```python
from build123d import *

# Parameters (mm, degrees)
ESBO_O1_W                = 22
ESBO_O1_H                = 36
RESSALTO_EXTRUS_O1_DEPTH = 110
CASCA1_T                 = -2
ESBO_O2_R                = 5
CORTE_EXTRUS_O1_DEPTH    = 1000
ESBO_O3_R                = 2.75
CORTE_EXTRUS_O2_DEPTH    = 29


with BuildPart() as part:
    # Esboço1 → Ressalto-extrusão1 (new body)
    with BuildSketch(Plane.XY):
        with Locations((0, 18)):
            Rectangle(ESBO_O1_W, ESBO_O1_H)
    extrude(amount=RESSALTO_EXTRUS_O1_DEPTH)

    # Casca1
    casca1_openings = [part.faces().sort_by_distance(p)[0] for p in [
        (0, 18, 0),
    ]]
    offset(amount=CASCA1_T, openings=casca1_openings, kind=Kind.INTERSECTION)

    # Esboço2 → Corte-extrusão1 (cut)
    with BuildSketch(Plane(origin=(0, 0, 0), x_dir=(-1, 0, 0), z_dir=(0, -1, 0))):
        with Locations(Location((0, -20, 0), (0, 0, 90))):
            Circle(ESBO_O2_R)
        with Locations(Location((0, -40, 0), (0, 0, 90))):
            Circle(ESBO_O2_R)
        with Locations(Location((0, -60, 0), (0, 0, 90))):
            Circle(ESBO_O2_R)
        with Locations(Location((0, -80, 0), (0, 0, 90))):
            Circle(ESBO_O2_R)
    extrude(amount=-CORTE_EXTRUS_O1_DEPTH, mode=Mode.SUBTRACT)

    # Esboço3 → Corte-extrusão2 (cut)
    with BuildSketch(Plane(origin=(11, 0, 0), x_dir=(0, 0, -1), z_dir=(1, 0, 0))):
        with Locations(Location((-90, 18, 0), (0, 0, 90))):
            Circle(ESBO_O3_R)
    extrude(amount=-CORTE_EXTRUS_O2_DEPTH, mode=Mode.SUBTRACT)


solid = part.part
```
Source: CAD feature listing. Evaluate the final solid. Frame: model axes, mm. A direction names the side the tool comes from. Give positions to 0.01 mm unless a question says otherwise; leave off trailing zeros. Loops run counter-clockwise (first coordinate to the right, second up) from the corner with the lowest first, then second, coordinate; pieces in that order, holes last. Notation, with made-up numbers: M 14.5,82 L 43.5,82 A30 ccw 43.5,114 Z; hole C -36,41.5 d6. An arc over 180 degrees is marked long. Put each result on its own line as item: value.
Q1. Section D-D (y = 6). Return the cut outline in (x, z).
Response values:
outline: M -11,0 L -9,0 L -9,108 L 9,108 L 9,0 L 11,0 L 11,110 L -11,110 Z
Q2. Reachability of faces 3 (the flat face through (0, 18, 108)), 4 (the cylindrical face through (-9.986, 17.404, 87.315)) from +Z, -Z, +X, -X, +Y, -Y: full face, straight path, thin tool, end or side. Return the list, or none.
Response values:
face 3: -Z
face 4: +X, -X
Q3. Section B-B (y = 18). Return the cut outline in (x, z).
Response values:
outline: M -11,0 L -9,0 L -9,87.25 L -11,87.25 Z; M -11,92.75 L -9,92.75 L -9,108 L 9,108 L 9,92.75 L 11,92.75 L 11,110 L -11,110 Z; M 9,0 L 11,0 L 11,87.25 L 9,87.25 Z
Q4. Section A-A (z = 90). Return the cut outline in (x, y), and give its area (3 significant figures).
Response values:
outline: M -11,0 L 11,0 L 11,15.25 L 9,15.25 L 9,2 L -9,2 L -9,15.25 L -11,15.25 Z; M -11,20.75 L -9,20.75 L -9,34 L 9,34 L 9,20.75 L 11,20.75 L 11,36 L -11,36 Z
area: 194 mm²
Q5. Pin query (flat end, axial travel): P1, Ø5.5, axis at x = 0, y = 13, coming from the -Z side. Return the tip coordinate at first contact, or that it passes through.
Response values:
P1: stops at z = 108
Q6. Line query: probe 1 along X at (y, z) = (25, 88); probe 2 along Y at (x, z) = (-8, 68); probe 3 along Z at (x, y) = (-8.5, 5). Output: solid intervals per line, ascending. Write a range as [from, to].
Response values:
probe 1: x = [-11, -9], [9, 11]
probe 2: y = [0, 2], [34, 36]
probe 3: z = [108, 110]
Q7. Section C-C (z = 71). Return the cut outline in (x, y).
Response values:
outline: M -11,0 L 11,0 L 11,36 L -11,36 Z; hole M -9,2 L 9,2 L 9,34 L -9,34 Z
Q8. Mould query, pull axis Y, two halves, no side actions, for faces 1 (the flat face through (-9, 18, 53)), 2 (the flat face through (0, 18, 110)). Classes: released by +Y, released by -Y, zero draft, split by the parting line, or undercut.
Response values:
face 1: undercut
face 2: zero draft
